Autodesk Inventor part; units mm, degrees
ref_plane "Plan YZ" through (0, 0, 0) normal (1, 0, 0) x (0, 1, 0)
ref_plane "Plan XZ" through (0, 0, 0) normal (0, 1, 0) x (-1, 0, 0)
ref_plane "Plan XY" through (0, 0, 0) normal (0, 0, 1) x (1, 0, 0)
sketch "Esquisse1" plane through (0, 0, 0) normal (0, 0, 1) x (1, 0, 0)
  line L0 (-125, -100) -> (125, -100)
  line L1 (125, -100) -> (125, 100)
  line L2 (125, 100) -> (-125, 100)
  line L3 (-125, 100) -> (-125, -100)
  line L4 (-125, -100) -> (125, 100) construction
  line L5 (125, -100) -> (-125, 100) construction
  point P0 (0, 0)
  dimension "d0" = 250
  dimension "d1" = 200
extrude "Extrusion1" add sketch "Esquisse1" along normal blind 59
sketch "Esquisse6" plane through (0, 0, 59) normal (0, 0, 1) x (1, 0, 0)
  line L0 (-120.7, -95.7) -> (120.7, -95.7)
  line L1 (120.7, -95.7) -> (120.7, 95.7)
  line L2 (120.7, 95.7) -> (-120.7, 95.7)
  line L3 (-120.7, 95.7) -> (-120.7, -95.7)
  line L4 (-120.7, -95.7) -> (120.7, 95.7) construction
  line L5 (120.7, -95.7) -> (-120.7, 95.7) construction
  line L6 (125, 100) -> (-125, 100)
  line L7 (125, -100) -> (125, 100)
  point P0 (0, 0)
  dimension "d4" = 4.3
  dimension "d5" = 4.3
extrude "Extrusion2" cut sketch "Esquisse6" against normal blind 57
sketch "Esquisse7" plane through (0, 0, 59) normal (0, 0, 1) x (1, 0, 0)
  line L0 (-121.7, -96.7) -> (121.7, -96.7)
  line L1 (121.7, -96.7) -> (121.7, 96.7)
  line L2 (121.7, 96.7) -> (-121.7, 96.7)
  line L3 (-121.7, 96.7) -> (-121.7, -96.7)
  line L4 (-121.7, -96.7) -> (121.7, 96.7) construction
  line L5 (121.7, -96.7) -> (-121.7, 96.7) construction
  line L6 (125, 100) -> (-125, 100)
  line L7 (125, -100) -> (125, 100)
  point P0 (0, 0)
  dimension "d8" = 3.3
  dimension "d9" = 3.3
extrude "Extrusion3" cut sketch "Esquisse7" against normal blind 2
fillet "Congé1" radius 3 12 edges at (-120.7, 95.7, 29.5) (-121.7, 96.7, 58) (-125, 100, 29.5) (120.7, 95.7, 29.5) (121.7, 96.7, 58) (120.7, -95.7, 29.5) (121.7, -96.7, 58) (-121.7, -96.7, 58) (-120.7, -95.7, 29.5) (-125, -100, 29.5) (125, -100, 29.5) (125, 100, 29.5)
sketch "Esquisse9" plane through (0, 0, 2) normal (0, 0, 1) x (1, 0, 0)
  line L0 (118.7, -96.7) -> (-118.7, -96.7)
  line L1 (-121.7, -93.7) -> (-121.7, 93.7)
  circle A0 centre (-116.7, -91.7) radius 4
  line L2 (0, 0) -> (0, 94.7693)
  line L3 (0, 0) -> (-121.7, 0)
  circle A1 centre (-116.7, 91.7) radius 4
  circle A2 centre (116.7, -91.7) radius 4
  circle A3 centre (116.7, 91.7) radius 4
  dimension "d15" = 5
  dimension "d16" = 5
  dimension "d17" = 8
extrude "Extrusion4" add sketch "Esquisse9" along normal blind 55
sketch "Esquisse10" plane through (0, 0, 2) normal (0, 0, 1) x (1, 0, 0)
  line L0 (118.7, -96.7) -> (-118.7, -96.7)
  line L1 (121.7, 93.7) -> (121.7, -93.7)
  line L2 (-121.7, -93.7) -> (-121.7, 93.7)
  circle A0 centre (0, -91.7) radius 4
  line L3 (0, 0) -> (121.7, 0)
  circle A1 centre (0, 91.7) radius 4
  dimension "d20" = 5
  dimension "d21" = 243.4
  dimension "d22" = 121.7
  dimension "d23" = 8
extrude "Extrusion5" add sketch "Esquisse10" along normal blind 55
sketch "Esquisse14" plane through (0, 0, 2) normal (0, 0, 1) x (1, 0, 0)
  line L0 (-120.7, 91.7) -> (-120.7, -91.7)
  line L1 (-116.7, -95.7) -> (0, -95.7)
  line L2 (0, 95.7) -> (-116.7, 95.7)
  circle A0 centre (-115.7, 0) radius 4
  circle A1 centre (0, 91.7) radius 4
  line L3 (0, 0) -> (0, 91.7)
  circle A2 centre (115.7, 0) radius 4
  dimension "d45" = 5
  dimension "d46" = 191.4
  dimension "d47" = 95.7
  dimension "d48" = 8
extrude "Extrusion7" add sketch "Esquisse14" along normal blind 55 contours A0 | A2
sketch "Esquisse12" plane through (0, 91.7, 57) normal (0, 0, 1) x (1, 0, 0)
  circle A0 centre (0, 0) radius 4
  arc A1 (116.7, 4) -> (120.7, 0) centre (116.7, 0) ccw
  arc A2 (120.7, -183.4) -> (116.7, -187.4) centre (116.7, -183.4) ccw
  arc A3 (-120.7, 0) -> (-116.7, 4) centre (-116.7, 0) ccw
  circle A4 centre (0, -183.4) radius 4
  arc A5 (-116.7, -187.4) -> (-120.7, -183.4) centre (-116.7, -183.4) ccw
  circle A6 centre (-115.7, -91.7) radius 4
  circle A7 centre (115.7, -91.7) radius 4
  point P0 (0, -91.7)
  point P1 (0, 4)
  point P2 (0, -187.4)
hole "Perçage1" at (0, 91.7, 57) at (116.7, 91.7, 57) at (116.7, -91.7, 57) at (-116.7, 91.7, 57) at (0, -91.7, 57) at (-116.7, -91.7, 57) at (115.7, 0, 57) at (-115.7, 0, 57) direction (0, 0, -1) diameter 2.459 depth 20 tip angle 118
sketch "Esquisse13" plane through (-122, -100, 0) normal (0, -1, 0) x (1, 0, 0)
  line L0 (244, 59) -> (244, 0)
  line L1 (0, 59) -> (244, 59)
  line L2 (0, 0) -> (244, 0)
  circle A0 centre (154, 29.5) radius 12
  circle A1 centre (184, 29.5) radius 12
  circle A2 centre (214, 29.5) radius 12
  point P0 (122, 0)
  dimension "d33" = 30
  dimension "d34" = 30
  dimension "d35" = 30
  dimension "d36" = 59
  dimension "d37" = 29.5
  dimension "d38" = 29.5
  dimension "d39" = 29.5
  dimension "d40" = 24
  dimension "d41" = 24
  dimension "d42" = 24
extrude "Extrusion6" cut sketch "Esquisse13" against normal blind 10
properties part number "Box" material "."
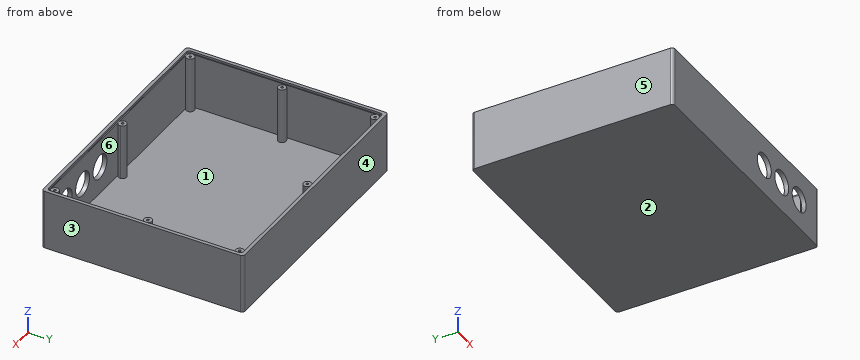
Read the model definition and answer for the solid it produces. Units are mm, in the model's axes. Face numbers are marked on the shaded views. A direction names the side the tool comes from. Round coordinates to 2 decimals unless told otherwise and drop trailing zeros. Loops run counter-clockwise (first coordinate to the right, second up) from the corner with the lowest first, then second, coordinate; pieces in that order, holes last.
Q1. Section D-D on y = 21.5 is taken. Write down the section's boundary in (x, z).
Q2. Each of these flat-tipped pins is pushed along its axis until it touches: pin 1 (2 mm diameter, centred on x = -119.5, y = -94, fed in from +Z); pin 2 (12 mm diameter, centred on x = 22.5, y = 55.5, fed in from +Z); pin 3 (21.5 mm diameter, centred on x = 62, z = 29.5, fed in from -Y). Where does it stop, or does it pass through?
Q3. Determine the mould class of the marked faces 3, 4, 5 and 6 for opening direction X: released by +X, released by -X, zero draft, split by the parting line, or undercut.
Q4. Which of the six approach directions +Z, -Z, +X, -X, +Y, -Y give full straight-line access (tool end or side, diameter ignored) to the marked faces 1 and 2?
Q5. Consider probe 1 along X at (y, z) = (-96, 29); probe 2 along X at (y, z) = (-76, 42); probe 3 along Y at (x, z) = (35.5, 10.5). Determine where each line is inside the solid, lowest interval first.
Q6. Section C-C on x = -60 is taken. Write down the section's boundary in (y, z), and give its area (3 significant figures).
Q7. Section A-A on x = 32 is taken. Write down the section's boundary in (y, z).
Output:
1. outline: (-125, 0) - (125, 0) - (125, 59) - (121.7, 59) - (121.7, 57) - (120.7, 57) - (120.7, 2) - (-120.7, 2) - (-120.7, 57) - (-121.7, 57) - (-121.7, 59) - (-125, 59) - close
2. pin 1: stops at z = 57
2. pin 2: stops at z = 2
2. pin 3: stops at y = 95.7
3. face 3: released by +X
3. face 4: zero draft
3. face 5: released by -X
3. face 6: undercut
4. face 1: +Z
4. face 2: -Z, +X, -X, +Y, -Y
5. probe 1: x = -125 to 20.01, 43.99 to 50.01, 73.99 to 80.01, 103.99 to 125
5. probe 2: x = -125 to -120.7, 120.7 to 125
5. probe 3: y = -100 to -95.7, 95.7 to 100
6. outline: (-100, 0) - (100, 0) - (100, 59) - (96.7, 59) - (96.7, 57) - (95.7, 57) - (95.7, 2) - (-95.7, 2) - (-95.7, 57) - (-96.7, 57) - (-96.7, 59) - (-100, 59) - close
6. area: 886 mm2
7. outline: (-100, 0) - (100, 0) - (100, 59) - (96.7, 59) - (96.7, 57) - (95.7, 57) - (95.7, 2) - (-95.7, 2) - (-95.7, 17.5) - (-100, 17.5) - close; (-100, 41.5) - (-95.7, 41.5) - (-95.7, 57) - (-96.7, 57) - (-96.7, 59) - (-100, 59) - close
